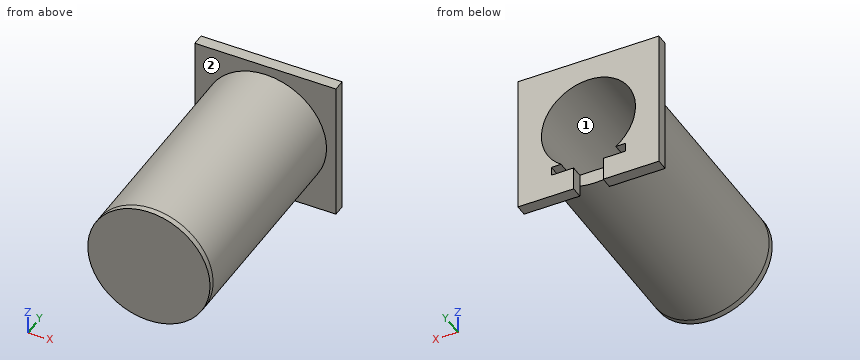
Autodesk Inventor part; units mm, degrees
ref_plane "YZ Plane" through (0, 0, 0) normal (1, 0, 0) x (0, 1, 0)
ref_plane "XZ Plane" through (0, 0, 0) normal (0, 1, 0) x (-1, 0, 0)
ref_plane "XY Plane" through (0, 0, 0) normal (0, 0, 1) x (1, 0, 0)
sketch "Sketch1" plane through (0, 0, 0) normal (0, 1, 0) x (-1, 0, 0)
  circle A0 centre (0, 0) radius 16.51
  dimension "d0" = 33.02
extrude "Extrusion1" add sketch "Sketch1" along normal blind 58.42
sketch "Sketch3" plane through (0, 58.42, 0) normal (0, 1, 0) x (1, 0, 0)
  line L0 (-19.05, 19.05) -> (19.05, 19.05)
  line L1 (19.05, 19.05) -> (19.05, -19.05)
  line L2 (19.05, -19.05) -> (-19.05, -19.05)
  line L3 (-19.05, -19.05) -> (-19.05, 19.05)
  point P0 (0, 0)
  point P1 (19.05, 0)
  point P2 (0, 19.05)
  dimension "d8" = 38.1
  dimension "d9" = 38.1
extrude "Extrusion3" add sketch "Sketch3" along normal blind 3.175
sketch "Sketch4" plane through (0, 61.595, 0) normal (0, 1, 0) x (1, 0, 0)
  circle A0 centre (0, 0) radius 12.7
  line L0 (-10, 12.7) -> (10, 12.7)
  line L1 (10, 12.7) -> (10, 10.3187)
  line L2 (10, 10.3187) -> (-10, 10.3187)
  line L3 (-10, 10.3187) -> (-10, 12.7)
  point P0 (-12.7, 0)
  point P1 (12.7, 0)
  point P2 (0, 12.7)
  point P3 (-7.4036, 10.3187)
  point P4 (7.4036, 10.3187)
  dimension "d12" = 25.4
  dimension "d13" = 20
  dimension "d14" = 2.3813
extrude "Extrusion4" cut sketch "Sketch4" against normal blind 61.9125
sketch "Sketch5" plane through (19.05, 58.42, -19.05) normal (0, 0, -1) x (-1, 0, 0)
  line L0 (15.05, 0) -> (23.05, 0)
  line L1 (23.05, 0) -> (23.05, 3.175)
  line L2 (23.05, 3.175) -> (15.05, 3.175)
  line L3 (15.05, 3.175) -> (15.05, 0)
  line L4 (0, 0) -> (0, 3.175)
  line L5 (0, 3.175) -> (38.1, 3.175)
  point P0 (19.05, -58.42)
  point P1 (19.05, 1.5875)
  point P2 (23.05, 1.5875)
  point P3 (19.05, 3.175)
  dimension "d17" = 8
  dimension "d18" = 3.175
  dimension "d20" = 19.05
  dimension "d21" = 0
extrude "Extrusion5" cut sketch "Sketch5" against normal blind 12.7
sketch "Sketch6" plane through (0, 0, 0) normal (0, -1, 0) x (1, 0, 0)
  arc A0 (7.4036, -10.3187) -> (-7.4036, -10.3187) centre (0, 0) ccw
  circle A1 centre (0, 0) radius 16.51
extrude "Extrusion6" add sketch "Sketch6" along normal blind 1.5875
properties part number "WaterBucket2"
Input: part model. Units: mm. Frame: model coordinates. Face numbers are marked on the shaded views. Coordinates: 2 decimals unless noted, no trailing zeros. Write each loop counter-clockwise with the first axis right and the second up, starting at its lowest first coordinate (ties: lowest second). Pieces come first, ordered by that corner, then holes.
1) Pin query (flat end, axial travel): pin 1 Ø0.7 at (y, z) = (41, -11) entering from +X; pin 2 Ø2.5 at (y, z) = (25.5, -11.5) entering from -X; pin 3 Ø10 at (x, y) = (4, 18) entering from -Z. Return the tip coordinate at first contact, or that it passes through.
2) Section A-A on y = 51. Output: boundary loops of the cut face in (x, z), and give its area (3 significant figures).
3) Mould query, pull axis X, two halves, no side actions, for the marked faces 1 and 2. Classes: pulls with the +X half, pulls with the -X half, needs draft (parallel to the pull), parting line crosses it, or undercut.
4) Material intervals for line 1 along X through (y, z) = (22, 0); line 2 along Y through (x, z) = (-8, -14.5) (3 decimals), sorted ascending.
Check result:
1. pin 1: stops at x = 12.62
1. pin 2: stops at x = -12.94
1. pin 3: stops at z = -16.51
2. outline: circle Ø33.02 at (0, 0); hole (-10, -12.7) - (10, -12.7) - (10, -10.32) - (7.4, -10.32) arc R12.7 ccw (long way) to (-7.4, -10.32) - (-10, -10.32) - close
2. area: 326 mm2
3. face 1: undercut
3. face 2: needs draft
4. line 1: x = -16.51 to -12.7, 12.7 to 16.51
4. line 2: y = 58.42 to 61.595
